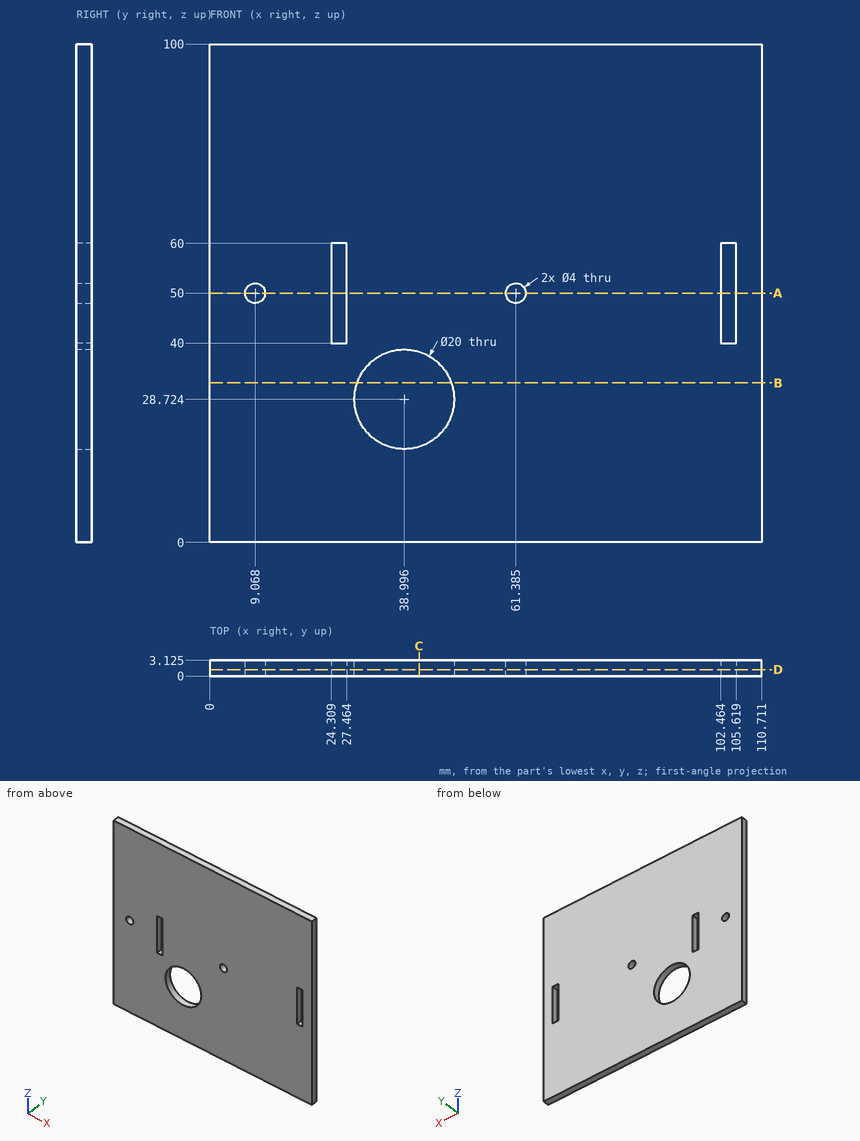
Input: dimensioned drawing with shaded views. Units: mm. Origin: part minimum x, y, z. Coordinates: 2 decimals unless noted, no trailing zeros. Loops run counter-clockwise (first coordinate to the right, second up) from the corner with the lowest first, then second, coordinate; pieces in that order, holes last.
Q1. Section A-A, the plane z = 50. Return the cut outline in (x, y) (1 decimal).
Results are:
outline: (0, 0) - (7.1, 0) - (7.1, 3.1) - (0, 3.1) - close; (11.1, 0) - (24.3, 0) - (24.3, 3.1) - (11.1, 3.1) - close; (27.5, 0) - (59.4, 0) - (59.4, 3.1) - (27.5, 3.1) - close; (63.4, 0) - (102.5, 0) - (102.5, 3.1) - (63.4, 3.1) - close; (105.6, 0) - (110.7, 0) - (110.7, 3.1) - (105.6, 3.1) - close
Q2. Section D-D, the plane y = 1.3. Return the cut outline in (x, z) (1 decimal).
Results are:
outline: (0, 0) - (110.7, 0) - (110.7, 100) - (0, 100) - close; hole circle Ø4 at (9.1, 50); hole (24.3, 40) - (27.5, 40) - (27.5, 60) - (24.3, 60) - close; hole circle Ø20 at (39, 28.7); hole circle Ø4 at (61.4, 50); hole (102.5, 40) - (105.6, 40) - (105.6, 60) - (102.5, 60) - close
Q3. Line query: line 1 along X through (y, z) = (2.5, 43); line 2 along X through (y, z) = (1.6, 50) (1 decimal); line 3 along Z through (x, y) = (26, 2.7). Output: solid intervals per line, ascending.
Results are:
line 1: x = 0 to 24.31, 27.46 to 102.46, 105.62 to 110.71
line 2: x = 0 to 7.1, 11.1 to 24.3, 27.5 to 59.4, 63.4 to 102.5, 105.6 to 110.7
line 3: z = 0 to 40, 60 to 100
Q4. Section B-B, the plane z = 32. Return the cut outline in (x, y) (1 decimal), and give its area (3 significant figures).
Results are:
outline: (0, 0) - (29.5, 0) - (29.5, 3.1) - (0, 3.1) - close; (48.4, 0) - (110.7, 0) - (110.7, 3.1) - (48.4, 3.1) - close
area: 287 mm2
Q5. Section C-C, the plane x = 42. Return the cut outline in (y, z) (1 decimal).
Results are:
outline: (0, 0) - (3.1, 0) - (3.1, 19.2) - (0, 19.2) - close; (0, 38.3) - (3.1, 38.3) - (3.1, 100) - (0, 100) - close
